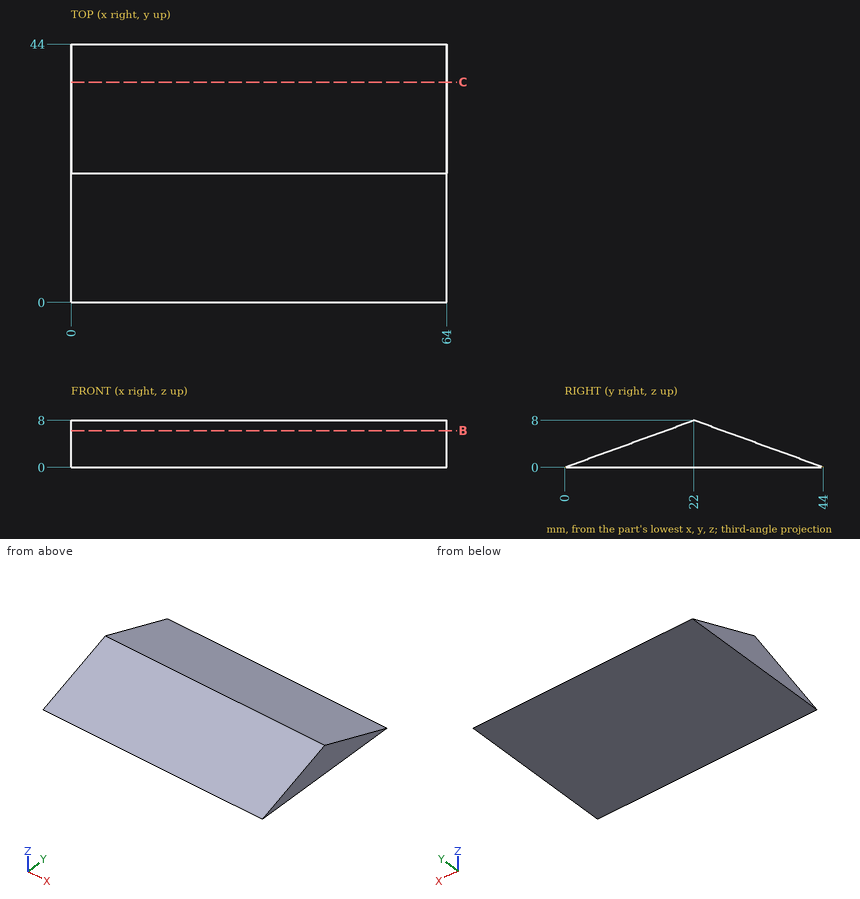
Check sheet for the drawn part. Datum: minimum x, y, z corner. Units: mm. Round coordinates to 2 decimals unless told otherwise and drop trailing zeros. Loops run counter-clockwise (first coordinate to the right, second up) from the corner with the lowest first, then second, coordinate; pieces in that order, holes last. Notation, with made-up numbers: (14, 64) - (48, 64) arc R24 ccw to (48, 91) - close; hole circle Ø10 at (-3, 3). An arc over 180 degrees is marked (long way). Write item = value, one per line. Start each with the question number.
1. Section check C-C on y = 37.5. Enter the section's corners in (x, z).
2. Depth check by flat-ended pin: pin 1 (1 mm diameter, centred on x = 38, y = 17.5, fed in from +Z). Enter the tip coordinate at first touch or a pass-through.
3. Thickness scan on line 1 (Z direction, x = 57.5, y = 21.5); line 2 (Z direction, x = 47.5, y = 10.5). Record the ranges inside material, lowest first.
4. Section check B-B on z = 6.25. Enter the section's corners in (x, y).
Working result:
q1.outline = (0, 0) - (64, 0) - (64, 2.36) - (0, 2.36) - close
q2.pin_1 = 6.55
q3.line_1 = 0 to 7.82
q3.line_2 = 0 to 3.82
q4.outline = (0, 17.19) - (64, 17.19) - (64, 26.81) - (0, 26.81) - close
